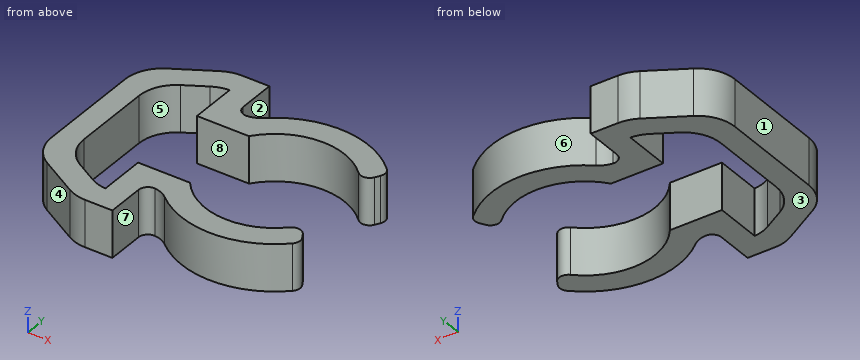
```python
from build123d import *

# Parameters (mm, degrees)
F1_DEPTH     = 6.35
F2_T1_DEPTH  = 6.35
F2_T3_DEPTH  = 6.35
F2_T5_DEPTH  = 6.35
F2_T7_DEPTH  = 6.35
F2_T9_DEPTH  = 13.1559094878
F2_T11_DEPTH = 21.0146968374
F2_T13_DEPTH = 21.0146968374
F2_T15_DEPTH = 13.1559094878
F3_R         = 3.175
F4_R         = 1.27
F5_R         = 1.27


# Not quite as in the source:
# - a fillet or chamfer that OpenCascade refuses, or shapes differently, is made with other operations: its cross-section is extruded or revolved along the edge and cut away or added


with BuildPart() as f1:
    # F0 (on Top) → F1 (new body)
    with BuildSketch(Plane.XY):
        with BuildLine():
            ThreePointArc((7.7709057387, -5.3975), (0.1961534845, -9.4594664786), (-7.5404746038, -5.715))
            Line((-7.5404746038, -5.715), (-14.605, -5.715))
            Line((-14.605, -5.715), (-14.605, -12.065))
            Line((-14.605, -12.065), (-15.659261314, -12.065))
            Line((-15.659261314, -12.065), (-22.225, -8.2742690022))
            Line((-22.225, -8.2742690022), (-22.225, 8.2742690022))
            Line((-22.225, 8.2742690022), (-15.659261314, 12.065))
            Line((-15.659261314, 12.065), (-14.605, 12.065))
            Line((-14.605, 12.065), (-14.605, 5.715))
            Line((-14.605, 5.715), (-7.5404746038, 5.715))
            ThreePointArc((-7.5404746038, 5.715), (0.1961534845, 9.4594664786), (7.7709057387, 5.3975))
            Line((7.7709057387, 5.3975), (9.5126338349, 8.4142615555))
            ThreePointArc((9.5126338349, 8.4142615555), (0.3250359785, 12.6958399333), (-9.0696141042, 8.89))
            Line((-9.0696141042, 8.89), (-11.43, 8.89))
            Line((-11.43, 8.89), (-11.43, 15.24))
            Line((-11.43, 15.24), (-16.51, 15.24))
            Line((-16.51, 15.24), (-25.4, 10.1073561069))
            Line((-25.4, 10.1073561069), (-25.4, -10.1073561069))
            Line((-25.4, -10.1073561069), (-16.51, -15.24))
            Line((-16.51, -15.24), (-11.43, -15.24))
            Line((-11.43, -15.24), (-11.43, -8.89))
            Line((-11.43, -8.89), (-9.0696141042, -8.89))
            ThreePointArc((-9.0696141042, -8.89), (0.3250359785, -12.6958399333), (9.5126338349, -8.4142615555))
            Line((9.5126338349, -8.4142615555), (7.7709057387, -5.3975))
        make_face()
    extrude(amount=F1_DEPTH)

    # F2: fillet of radius 5.08 on 8 edges, made by hand

    # F2_s2 → F2_t1 (join)
    with BuildSketch(Plane.XY):
        with BuildLine():
            ThreePointArc((-14.605, -12.065), (-15.7512023765, -11.857721614), (-16.8200610521, -11.3948119587))
            Line((-16.8200610521, -11.3948119587), (-15.659261314, -12.065))
            Line((-15.659261314, -12.065), (-14.605, -12.065))
        make_face()
    extrude(amount=F2_T1_DEPTH)

    # F2_s4 → F2_t3 (join)
    with BuildSketch(Plane.XY):
        with BuildLine():
            ThreePointArc((-19.685, -9.740738686), (-21.5444090512, -7.8813296347), (-22.225, -5.3413296347))
            Line((-22.225, -5.3413296347), (-22.225, -8.2742690022))
            Line((-22.225, -8.2742690022), (-19.685, -9.740738686))
        make_face()
    extrude(amount=F2_T3_DEPTH)

    # F2_s6 → F2_t5 (join)
    with BuildSketch(Plane.XY):
        with BuildLine():
            ThreePointArc((-22.225, 5.3413296347), (-21.5444090512, 7.8813296347), (-19.685, 9.740738686))
            Line((-19.685, 9.740738686), (-22.225, 8.2742690022))
            Line((-22.225, 8.2742690022), (-22.225, 5.3413296347))
        make_face()
    extrude(amount=F2_T5_DEPTH)

    # F2_s8 → F2_t7 (join)
    with BuildSketch(Plane.XY):
        with BuildLine():
            ThreePointArc((-16.8200610521, 11.3948119587), (-15.7512023765, 11.857721614), (-14.605, 12.065))
            Line((-14.605, 12.065), (-15.659261314, 12.065))
            Line((-15.659261314, 12.065), (-16.8200610521, 11.3948119587))
        make_face()
    extrude(amount=F2_T7_DEPTH)

    # F2_s10 → F2_t9 (cut)
    with BuildSketch(Plane.XY.offset(-3.4029547439)):
        with BuildLine():
            ThreePointArc((-15.1488181024, 15.24), (-16.4636188516, 15.0669031975), (-17.6888181024, 14.5594090512))
            Line((-17.6888181024, 14.5594090512), (-16.51, 15.24))
            Line((-16.51, 15.24), (-15.1488181024, 15.24))
        make_face()
    extrude(amount=F2_T9_DEPTH, mode=Mode.SUBTRACT)

    # F2_s12 → F2_t11 (cut)
    with BuildSketch(Plane.XY.offset(-7.3323484187)):
        with BuildLine():
            ThreePointArc((-25.4, 7.1744167394), (-24.7194090512, 9.7144167394), (-22.86, 11.5738257906))
            Line((-22.86, 11.5738257906), (-25.4, 10.1073561069))
            Line((-25.4, 10.1073561069), (-25.4, 7.1744167394))
        make_face()
    extrude(amount=F2_T11_DEPTH, mode=Mode.SUBTRACT)

    # F2_s14 → F2_t13 (cut)
    with BuildSketch(Plane.XY.offset(-7.3323484187)):
        with BuildLine():
            ThreePointArc((-22.86, -11.5738257906), (-24.7194090512, -9.7144167394), (-25.4, -7.1744167394))
            Line((-25.4, -7.1744167394), (-25.4, -10.1073561069))
            Line((-25.4, -10.1073561069), (-22.86, -11.5738257906))
        make_face()
    extrude(amount=F2_T13_DEPTH, mode=Mode.SUBTRACT)

    # F2_s16 → F2_t15 (cut)
    with BuildSketch(Plane.XY.offset(-3.4029547439)):
        with BuildLine():
            ThreePointArc((-15.1488181024, -15.24), (-16.4636188516, -15.0669031975), (-17.6888181024, -14.5594090512))
            Line((-17.6888181024, -14.5594090512), (-16.51, -15.24))
            Line((-16.51, -15.24), (-15.1488181024, -15.24))
        make_face()
    extrude(amount=F2_T15_DEPTH, mode=Mode.SUBTRACT)

    # F3
    f3_edges = [f1.edges().sort_by_distance(p)[0] for p in [
        (-9.069614, 8.89, 3.175),
        (-9.069614, -8.89, 3.175),
    ]]
    fillet(f3_edges, radius=F3_R)

    # F4
    f4_edges = [f1.edges().sort_by_distance(p)[0] for p in [
        (-11.43, -8.89, 3.175),
        (-11.43, 8.89, 3.175),
    ]]
    fillet(f4_edges, radius=F4_R)

    # F5
    f5_edges = [f1.edges().sort_by_distance(p)[0] for p in [
        (7.770906, -5.3975, 3.175),
        (9.512634, -8.414262, 3.175),
        (9.512634, 8.414262, 3.175),
        (7.770906, 5.3975, 3.175),
    ]]
    fillet(f5_edges, radius=F5_R)


solid = f1.part
```
For this review, take the finished solid that the model builds, in its own axes (mm). Face numbers are marked on the shaded views. A direction names the side the tool comes from. Give positions to 0.01 mm unless a question says otherwise; leave off trailing zeros. Write each loop counter-clockwise with the first axis right and the second up, starting at its lowest first coordinate (ties: lowest second). Pieces come first, ordered by that corner, then holes.
Item 1: Take a section at A-A (y = -11). Give the boundary of the cut face in (x, z) (3 decimals), and give its area (3 significant figures).
Item 2: Wall thickness on probe 1 along Y at (x, z) = (-11.5, 5.5) (3 decimals); probe 2 along X at (y, z) = (7.5, 3.5) (3 decimals); probe 3 along X at (y, z) = (-11.5, 1.5) (3 decimals): over which ranges is each line inside the solid? List them lowest first.
Item 3: The part is to be moulded in two halves that separate along X. For the marked faces 1, 2 and 3, say which applies: +X half, -X half, draft (parallel to the pull), parting line (faces both ways), or undercut.
Item 4: Machinability: for the marked faces 4, 5, 6, 7 and 8, which of the approach directions +Z, -Z, +X, -X, +Y, -Y give a long, thin tool a straight path to every point of the face, cutting with its end or side? Answer none if there is none.
Item 5: Take a section at C-C (y = 3). Give the boundary of the cut face in (x, z) (3 decimals).
Item 6: Take a section at B-B (x = -16). Give the boundary of the cut face in (y, z).
Item 7: Insertion check: P1, Ø1.5, axis at y = 12.5, z = 2, coming from the +X side; P2, Ø6, axis at x = -17, y = -0.5, coming from the +Z side; P3, Ø2, axis at y = 8.5, z = 4, coming from the -X side; P4, Ø3, axis at y = -1, z = 3, coming from the +X side (3 decimals). Each pin has a flat end and moves straight along its axis. Give the tip position at first contact, or say it passes through.
Item 8: Take a section at D-D (x = -6.5). Give the boundary of the cut face in (y, z).
Established:
1. outline: (-23.662, 0) - (-17.504, 0) - (-17.504, 6.35) - (-23.662, 6.35) - close; (-14.605, 0) - (-11.43, 0) - (-11.43, 6.35) - (-14.605, 6.35) - close; (-6.347, 0) - (6.347, 0) - (6.347, 6.35) - (-6.347, 6.35) - close
1. area: 140 mm2
2. probe 1: y = -15.24 to -5.715, 5.715 to 15.24
2. probe 2: x = -25.39 to -21.744, -14.605 to -5.768, 5.768 to 8.985
2. probe 3: x = -22.984 to -16.628, -14.605 to -11.43, -5.389 to 5.389
3. face 1: -X half
3. face 2: undercut
3. face 3: draft
4. face 4: +Z, -Z, -X, -Y
4. face 5: +Z, -Z
4. face 6: +Z, -Z, +Y
4. face 7: +Z, -Z, -Y
4. face 8: +Z, -Z, +X
5. outline: (-25.4, 0) - (-22.225, 0) - (-22.225, 6.35) - (-25.4, 6.35) - close
6. outline: (-15.17, 0) - (-11.78, 0) - (-11.78, 6.35) - (-15.17, 6.35) - close; (11.78, 0) - (15.17, 0) - (15.17, 6.35) - (11.78, 6.35) - close
7. P1: stops at x = 4.82
7. P2: passes through
7. P3: stops at x = -25.39
7. P4: stops at x = -22.225
8. outline: (-10.91, 0) - (-6.88, 0) - (-6.88, 6.35) - (-10.91, 6.35) - close; (6.88, 0) - (10.91, 0) - (10.91, 6.35) - (6.88, 6.35) - close
